Read the model definition and answer for the solid it produces. Units are mm, in the model's axes. Face numbers are marked on the shaded views. A direction names the side the tool comes from. Coordinates: 2 decimals unless noted, no trailing zeros. Order: outer loops, then holes, each group sorted by start corner. A loop starts at its lowest first (then second) coordinate and runs counter-clockwise, first axis right, second up. Notation, with made-up numbers: M 69,49.5 L 87,49.5 A7 ccw 87,58.5 Z; hole C 5,3 d6. An arc over 180 degrees is marked long. One line per question, with ' | ' between items. Start each with the question number.
1) Find section B-B, the plane x = -0.25. Write down the section's boundary in (y, z), plus the area to 3 significant figures.
2) Given P1, Ø1.5, axis at x = 2.5, z = 8, coming from the -Y side; P2, Ø2, axis at x = -4, z = 7, coming from the -Y side; P3, Ø1.3, axis at y = -1, z = 13, coming from the +X side; P4, Ø3, axis at x = 0, y = 0, coming from the +Z side, each flat-ended and moving along its own axis, determine where each tip first touches the part or whether it passes through.
3) The mould has two halves that part along X. Classify the marked faces 4, 5 and 6: +X half, -X half, draft (parallel to the pull), parting line (faces both ways), or undercut.
4) A tool of negligible diameter and unlimited length cuts with its end or side. For the marked faces 1, 2 and 3, from which of +Z, -Z, +X, -X, +Y, -Y can it reach the whole face along a straight path? Write none if from no direction.
5) Consider probe 1 along Z at (x, y) = (-2.5, -2.75); probe 2 along Z at (x, y) = (2.5, 1); probe 3 along X at (y, z) = (-0.75, 9.25). Determine where each line is inside the solid, lowest interval first.
6) Find section C-C, the plane z = 1.5. Write down the section's boundary in (x, y).
7) Find section D-D, the plane z = 12.5. Write down the section's boundary in (x, y).
8) Find section A-A, the plane y = 1. Write down the section's boundary in (x, z), plus the area to 3 significant figures.
from build123d import *

# Parameters (mm, degrees)
SKETCH048_R       = 1.7
PAD023_DEPTH      = 17
BOX_W             = 6
BOX_H             = 20
BOX_DEPTH         = 2.55
BOX001_W          = 10
BOX001_H          = 10
BOX001_DEPTH      = 30
CYLINDER_R        = 1.7
CYLINDER_DEPTH    = 10
CYLINDER001_R     = 1.7
CYLINDER001_DEPTH = 11


with BuildPart() as part:
    # Sketch048 → Pad023 (new body)
    with BuildSketch(Plane.XY):
        Polygon((0, 4.5), (-8.5, -4), (8.5, -4), align=None)
        Circle(SKETCH048_R, mode=Mode.SUBTRACT)
    extrude(amount=PAD023_DEPTH)

    # Box → Box (cut)
    with BuildSketch(Plane(origin=(-3, -6, 12), x_dir=(1, 0, 0), z_dir=(0, 0, 1))):
        with Locations((3, 10)):
            Rectangle(BOX_W, BOX_H)
    extrude(amount=BOX_DEPTH, mode=Mode.SUBTRACT)

    # Box001 → Box001 (cut)
    with BuildSketch(Plane(origin=(0, -12, -20), x_dir=(0.707107, 0.707107, 0), z_dir=(0, 0, 1))):
        with Locations((5, 5)):
            Rectangle(BOX001_W, BOX001_H)
    extrude(amount=BOX001_DEPTH, mode=Mode.SUBTRACT)

    # Cylinder → Cylinder (cut)
    with BuildSketch(Plane(origin=(2, -4, 5), x_dir=(-0.707107, 0.707107, 0), z_dir=(0.707107, 0.707107, 0))):
        Circle(CYLINDER_R)
    extrude(amount=CYLINDER_DEPTH, mode=Mode.SUBTRACT)

    # Cylinder001 → Cylinder001 (cut)
    with BuildSketch(Plane(origin=(-10, 4, 4), x_dir=(0.707107, 0.707107, 0), z_dir=(0.707107, -0.707107, 0))):
        Circle(CYLINDER001_R)
    extrude(amount=CYLINDER001_DEPTH, mode=Mode.SUBTRACT)


solid = part.part
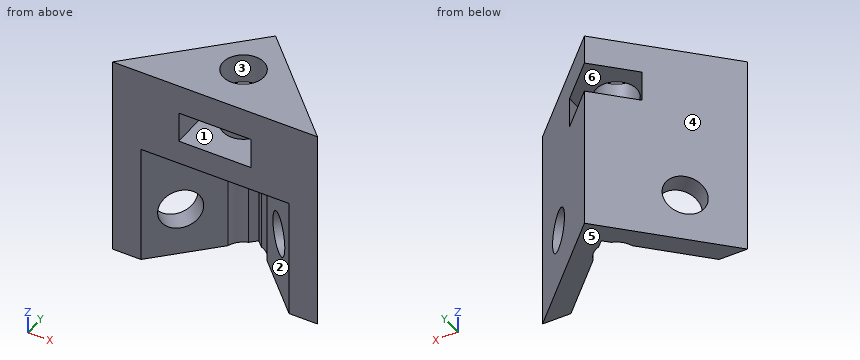
Report:
1) outline: M -4,10 L -1.68,10 L -1.68,12 L -4,12 Z; M -4,14.55 L -1.68,14.55 L -1.68,17 L -4,17 Z; M 1.68,10 L 1.89,10 L 1.89,0 L 4.25,0 L 4.25,12 L 1.68,12 Z; M 1.68,14.55 L 4.25,14.55 L 4.25,17 L 1.68,17 Z | area: 45.3 mm^2
2) P1: stops at y = -1.11 | P2: stops at y = -2.86 | P3: stops at x = 6.15 | P4: passes through
3) face 4: -X half | face 5: draft | face 6: undercut
4) face 1: +Y, -Y | face 2: -Z, -Y | face 3: +Z, -Z
5) probe 1: z = 10 to 12, 14.55 to 17 | probe 2: z = 0 to 12, 14.55 to 17 | probe 3: x = -5.25 to -2.89, 2.89 to 5.25
6) outline: M -8.5,-4 L -6.14,-4 L -1.62,0.53 A1.7 cw -0.53,1.62 L 0,2.14 L 0.53,1.62 A1.7 cw 1.62,0.53 L 6.14,-4 L 8.5,-4 L 0,4.5 Z
7) outline: M -8.5,-4 L -3,-4 L -3,1.5 Z; M 3,-4 L 8.5,-4 L 3,1.5 Z
8) outline: M -3.5,0 L -1.37,0 L -1.37,12 L -3,12 L -3,14.55 L -1.37,14.55 L -1.37,17 L -3.5,17 Z; M 1.37,0 L 3.5,0 L 3.5,17 L 1.37,17 L 1.37,14.55 L 3,14.55 L 3,12 L 1.37,12 Z | area: 64.0 mm^2
